```python
from build123d import *

# Parameters (mm, degrees)
SKETCH_1_R          = 2.55
EXTRUDE_1_DEPTH     = 7
SKETCH_3_R          = 2.55
EXTRUDE_2_DEPTH     = 7
EXTRUDE_3_DEPTH     = 11
SKETCH_5_R          = 2.55
EXTRUDE_4_DEPTH     = 3
EXTRUDE_START       = 7
SKETCH_6_R          = 7
SKETCH_6_R_2        = 2.55
EXTRUDE_5_DEPTH     = 7
SKETCH_7_R          = 1.3
CUT_EXTRUDE_1_DEPTH = 5
SKETCH_8_R          = 1.3
CUT_EXTRUDE_2_DEPTH = 5
SKETCH_9_R          = 5
CUT_EXTRUDE_3_DEPTH = 1.5
CUT_EXTRUDE_4_REACH = 38.718
FILLET_1_R          = 2


with BuildPart() as part:
    # Эскиз1 → Бобышка-Вытянуть1 (new body)
    with BuildSketch(Plane(origin=(0, 0, 0), x_dir=(1, 0, 0), z_dir=(0, 1, 0))):
        with BuildLine():
            Line((8.8, 25), (-16.8, 25))
            Line((-16.8, 25), (-16.8, -3))
            ThreePointArc((-16.8, -3), (-16.214213562, -4.414213562), (-14.8, -5))
            Line((-14.8, -5), (-13.979301231, -5))
            ThreePointArc((-13.979301231, -5), (-12.565087669, -5.585786438), (-11.979301231, -7))
            Line((-11.979301231, -7), (-11.979301231, -23))
            ThreePointArc((-11.979301231, -23), (-11.393514794, -24.414213562), (-9.979301231, -25))
            Line((-9.979301231, -25), (16.8, -25))
            Line((16.8, -25), (16.8, 17))
            Line((16.8, 17), (8.8, 25))
        make_face()
        with Locations(Location((4.8, 3.5, 0), (0, 0, 270))):
            Circle(SKETCH_1_R, mode=Mode.SUBTRACT)
        with Locations(Location((-3.489533647, -13.352791034, 0), (0, 0, 270))):
            Circle(SKETCH_1_R, mode=Mode.SUBTRACT)
    extrude(amount=EXTRUDE_1_DEPTH)

    # Эскиз3 → Бобышка-Вытянуть2 (add)
    with BuildSketch(Plane(origin=(0, 7, 0), x_dir=(1, 0, 0), z_dir=(0, 1, 0))):
        with BuildLine():
            Line((8.8, 25), (-16.8, 25))
            Line((-16.8, 25), (-16.8, -2.352791034))
            Line((-16.8, -2.352791034), (-3.489533647, -2.352791034))
            ThreePointArc((-3.489533647, -2.352791034), (4.288640946, -5.574616441), (7.510466353, -13.352791034))
            Line((7.510466353, -13.352791034), (7.510466353, -25))
            Line((7.510466353, -25), (16.8, -25))
            Line((16.8, -25), (16.8, 17))
            Line((16.8, 17), (8.8, 25))
        make_face()
        with Locations(Location((4.8, 3.5, 0), (0, 0, 270))):
            Circle(SKETCH_3_R, mode=Mode.SUBTRACT)
    extrude(amount=EXTRUDE_2_DEPTH)

    # Эскиз4 → Бобышка-Вытянуть3 (add)
    with BuildSketch(Plane(origin=(0, 14, 0), x_dir=(1, 0, 0), z_dir=(0, 1, 0))):
        with BuildLine():
            Line((8.800011647, 25), (-16.8, 25))
            Line((-16.8, 25), (-16.8, 14.5))
            Line((-16.8, 14.5), (4.8, 14.5))
            ThreePointArc((4.8, 14.5), (13.433239095, 10.316684145), (15.500011647, 0.948578679))
            Line((15.500011647, 0.948578679), (15.500011647, -25))
            Line((15.500011647, -25), (16.800011647, -25))
            Line((16.800011647, -25), (16.800011647, 17))
            Line((16.800011647, 17), (8.800011647, 25))
        make_face()
    extrude(amount=EXTRUDE_3_DEPTH)

    # Эскиз5 → Бобышка-Вытянуть4 (add)
    with BuildSketch(Plane(origin=(0, 25, 0), x_dir=(1, 0, 0), z_dir=(0, 1, 0))):
        with BuildLine():
            Line((8.8, 25), (-16.8, 25))
            Line((-16.8, 25), (-16.8, -3))
            ThreePointArc((-16.8, -3), (-16.214213562, -4.414213562), (-14.8, -5))
            Line((-14.8, -5), (-13.979301231, -5))
            ThreePointArc((-13.979301231, -5), (-12.565087669, -5.585786438), (-11.979301231, -7))
            Line((-11.979301231, -7), (-11.979301231, -17.343145751))
            ThreePointArc((-11.979301231, -17.343145751), (-9.736660544, -22.757359313), (-4.322446982, -25))
            Line((-4.322446982, -25), (16.8, -25))
            Line((16.8, -25), (16.8, 17))
            Line((16.8, 17), (8.8, 25))
        make_face()
        with Locations(Location((4.8, 3.5, 0), (0, 0, 270))):
            Circle(SKETCH_5_R, mode=Mode.SUBTRACT)
        with Locations(Location((-3.489533647, -13.352791034, 0), (0, 0, 270))):
            Circle(SKETCH_5_R, mode=Mode.SUBTRACT)
    extrude(amount=EXTRUDE_4_DEPTH)

    # Эскиз6 → Бобышка-Вытянуть5 (add)
    with BuildSketch(Plane.XZ.offset(-25).offset(EXTRUDE_START)):
        with Locations(Location((-3.489533647, 13.352791034, 0), (0, 0, 90))):
            Circle(SKETCH_6_R)
        with Locations(Location((-3.489533647, 13.352791034, 0), (0, 0, 90))):
            Circle(SKETCH_6_R_2, mode=Mode.SUBTRACT)
    extrude(amount=-EXTRUDE_5_DEPTH)

    # Эскиз7 → Вырез-Вытянуть1 (cut)
    with BuildSketch(Plane(origin=(0, 0, -25), x_dir=(-1, 0, 0), z_dir=(0, 0, -1))):
        with Locations((4, 13.75)):
            Circle(SKETCH_7_R)
    extrude(amount=-CUT_EXTRUDE_1_DEPTH, mode=Mode.SUBTRACT)

    # Эскиз8 → Вырез-Вытянуть2 (cut)
    with BuildSketch(Plane(origin=(16.8, 0, 0), x_dir=(0, 0, -1), z_dir=(1, 0, 0))):
        with Locations((-4, 7)):
            Circle(SKETCH_8_R)
    extrude(amount=-CUT_EXTRUDE_2_DEPTH, mode=Mode.SUBTRACT)

    # Эскиз9 → Вырез-Вытянуть3 (cut)
    with BuildSketch(Plane(origin=(0, 28, 0), x_dir=(1, 0, 0), z_dir=(0, 1, 0))):
        with Locations(Location((4.8, 3.5, 0), (0, 0, 270))):
            Circle(SKETCH_9_R)
        with Locations(Location((-3.489533647, -13.352791034, 0), (0, 0, 270))):
            Circle(SKETCH_9_R)
    extrude(amount=-CUT_EXTRUDE_3_DEPTH, mode=Mode.SUBTRACT)

    # Эскиз11 → Вырез-Вытянуть4 (cut, up to next)
    with BuildSketch(Plane(origin=(0, 7, 0), x_dir=(1, 0, 0), z_dir=(0, 1, 0)), mode=Mode.PRIVATE) as cut_extrude_4_sk1:
        with BuildLine():
            Line((-11.979301231, -17.343145751), (-11.979301231, -25))
            Line((-11.979301231, -25), (-4.322446982, -25))
            ThreePointArc((-4.322446982, -25), (-9.736660544, -22.757359313), (-11.979301231, -17.343145751))
        make_face()
    cut_extrude_4_tool1 = extrude(cut_extrude_4_sk1.sketch, amount=-CUT_EXTRUDE_4_REACH, mode=Mode.PRIVATE) & part.part
    add(cut_extrude_4_tool1.solids().sort_by_distance((-10.269005, 7, 23.289704))[0], mode=Mode.SUBTRACT)

    # Скругление1
    fillet_1_edges = [part.edges().sort_by_distance(p)[0] for p in [
        (-3.489533647, 25, 6.352791034),
    ]]
    fillet(fillet_1_edges, radius=FILLET_1_R)


solid = part.part
```
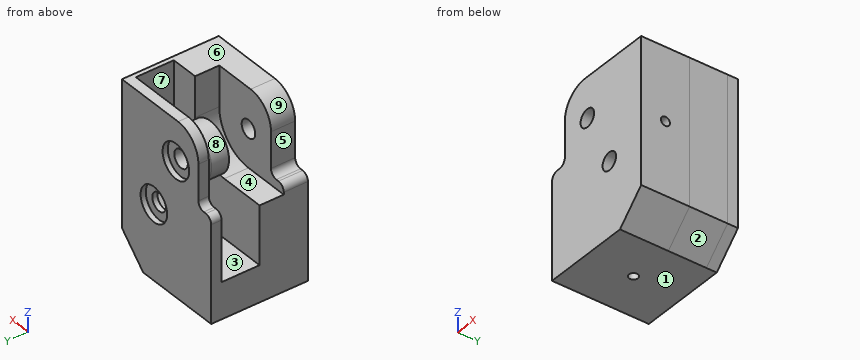
Check sheet for the modelled part. Datum: model origin and axes. Units: mm. Face numbers are marked on the shaded views. A direction names the side the tool comes from. Round coordinates to 2 decimals unless told otherwise and drop trailing zeros. Order: outer loops, then holes, each group sorted by start corner. A loop starts at its lowest first (then second) coordinate and runs counter-clockwise, first axis right, second up. Notation, with made-up numbers: M -13.5,23 L 24.5,23 A13 cw 24.5,30 Z; hole C 59,6.25 d9. An arc over 180 degrees is marked long. Answer in a Markdown table with one row per item.
(1) Material ranges on line 1 along Y through (x, z) = (1, -10); line 2 along X through (y, z) = (26.1, -3.5); line 3 along Y through (x, z) = (2.5, 20.5), recorded low to high. Write a range as from..to.
Findings:
| item | result |
|---|---|
| line 1 | y = 0..14, 25..28 |
| line 2 | x = -16.8..2.25, 7.35..16.8 |
| line 3 | y = 0..7, 25..28 |
(2) Section check B-B on y = 10.25. Record the boundary of the cut face in (x, z).
Findings:
| item | result |
|---|---|
| outline | M -16.8,-25 L 8.8,-25 L 16.8,-17 L 16.8,25 L 7.51,25 L 7.51,13.35 A11 cw -3.49,2.35 L -16.8,2.35 Z; hole C 4.8,-3.5 d5.1 |
(3) Draft check along X on the marked faces 6, 7, 8 and 9. Enter one of: +X half, -X half, draft (parallel to the pull), parting line (faces both ways), or undercut.
Findings:
| item | result |
|---|---|
| face 6 | draft |
| face 7 | undercut |
| face 8 | undercut |
| face 9 | -X half |
(4) Gauge pin test, flat ends, axial feed: pin 1 (1 mm diameter, centred on y = 23, z = -0.5, fed in from -X); pin 2 (0.9 mm diameter, centred on x = -14, y = 26.5, fed in from +Z); pin 3 (2 mm diameter, centred on x = -4, y = 13.75, fed in from -Z). Record the tip position at first contact, or that the pin passes through.
Findings:
| item | result |
|---|---|
| pin 1 | stops at x = 15.5 |
| pin 2 | stops at z = 5.05 |
| pin 3 | stops at z = -20 |
(5) Section check A-A on y = 25.75. Record the boundary of the cut face in (x, z), plus the area to 3 significant figures.
Findings:
| item | result |
|---|---|
| outline | M -16.8,-25 L 8.8,-25 L 16.8,-17 L 16.8,25 L -4.32,25 A7.66 ccw -11.98,17.34 L -11.98,7 A2 cw -13.98,5 L -14.8,5 A2 ccw -16.8,3 Z; hole C -3.49,13.35 d5.1; hole C 4.8,-3.5 d5.1 |
| area | 1,500 mm^2 |
(6) Set-up check for the marked faces 1, 2, 3, 4 and 5: record each of +Z, -Z, +X, -X, +Y, -Y from which the full face is reachable in a straight line by a thin tool's end or side.
Findings:
| item | result |
|---|---|
| face 1 | -Z, +X, -X, +Y, -Y |
| face 2 | -Z, +X, +Y, -Y |
| face 3 | -X |
| face 4 | +Z, -X |
| face 5 | +Z, -X, +Y, -Y |
